from build123d import *

# Parameters (mm, degrees)
SKETCH_1_R      = 2.5
EXTRUDE_1_DEPTH = 1


with BuildPart() as part:
    # 스케치1 → 보스-돌출1 (new body)
    with BuildSketch(Plane.XY):
        with BuildLine():
            Line((18.529028891, 5), (0, 5))
            ThreePointArc((0, 5), (-3.535533906, 3.535533906), (-5, 0))
            Line((-5, 0), (-5, -2.326474397))
            Line((-5, -2.326474397), (-1.043619368, -5.799632967))
            Line((-1.043619368, -5.799632967), (-1.043619368, -29.024920851))
            Line((-1.043619368, -29.024920851), (0.023324735, -29.024920851))
            ThreePointArc((0.023324735, -29.024920851), (4.304027875, -26.817883884), (6.134722324, -22.363224595))
            Line((6.134722324, -22.363224595), (6.134722324, -2.376138068))
            Line((6.134722324, -2.376138068), (17.489524427, -2.376138068))
            Line((17.489524427, -2.376138068), (18.529028891, 5))
        make_face()
        Circle(SKETCH_1_R, mode=Mode.SUBTRACT)
    extrude(amount=EXTRUDE_1_DEPTH)


solid = part.part
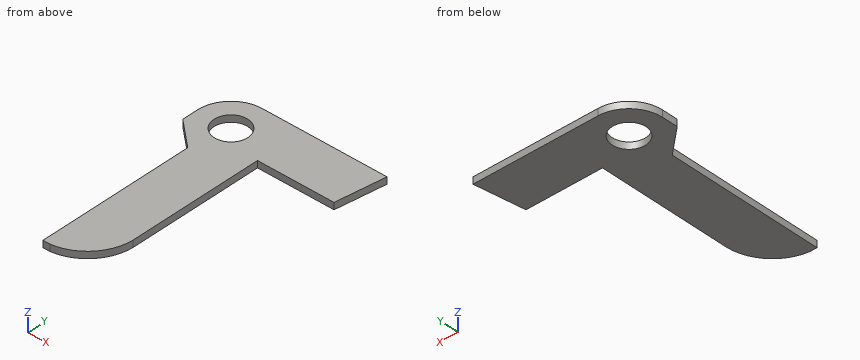
Source: CAD feature listing. Evaluate the final solid. Frame: model axes, mm. Round coordinates to 2 decimals unless told otherwise and drop trailing zeros. Loops run counter-clockwise (first coordinate to the right, second up) from the corner with the lowest first, then second, coordinate; pieces in that order, holes last. Notation, with made-up numbers: (66.25, 31) - (123.25, 31) arc R29 ccw to (123.25, 55) - close; hole circle Ø8 at (-35.5, -29). An arc over 180 degrees is marked (long way). Write item = value, one per line. Start each with the question number.
Item 1: Section query C-C on x = 9.5. Output: boundary loops of the cut face in (y, z).
Item 2: Section query A-A on z = 0.4. Output: boundary loops of the cut face in (x, y), plus the area to 3 significant figures.
Item 3: Material intervals for line 1 (Y direction, x = 0, z = 0.85); line 2 (X direction, y = -22, z = 0.4); line 3 (Y direction, x = 14.5, z = 0.95), sorted ascending.
Item 4: First-contact query: pin 1 Ø0.5 at (y, z) = (-20.5, 0.5) entering from -X; pin 2 Ø0.5 at (y, z) = (-11, 0.5) entering from +X; pin 3 Ø1.5 at (x, y) = (8, -19.5) entering from +Z. Flat tips, straight axial feed; report the tip coordinate or a pass-through.
Item 5: Section query B-B on y = -11.5. Output: boundary loops of the cut face in (x, z), plus the area to 3 significant figures.
Results list:
q1.outline = (-2.38, 0) - (5, 0) - (5, 1) - (-2.38, 1) - close
q2.outline = (-5, -2.33) - (-1.04, -5.8) - (-1.04, -29.02) - (0.02, -29.02) arc R6.98 ccw to (6.13, -22.36) - (6.13, -2.38) - (17.49, -2.38) - (18.53, 5) - (0, 5) arc R5 ccw to (-5, 0) - close; hole circle Ø5 at (0, 0)
q2.area = 333 mm²
q3.line_1 = -29.02 to -2.5, 2.5 to 5
q3.line_2 = -1.04 to 6.13
q3.line_3 = -2.38 to 5
q4.pin_1 = -1.04
q4.pin_2 = 6.13
q4.pin_3 = through
q5.outline = (-1.04, 0) - (6.13, 0) - (6.13, 1) - (-1.04, 1) - close
q5.area = 7.18 mm²
